```python
from build123d import *

# Parameters (mm, degrees)
F1_DEPTH = 40
F4_DEPTH = 22.7
F6_D     = 3
F6_DEPTH = 5
F6_TIP   = 0.9012909285


with BuildPart() as f1:
    # F0 (on Top) → F1 (new body)
    with BuildSketch(Plane.XY):
        Polygon((16.9819894888, 21.025), (-16.9819894888, 21.025), (-21.025, 16.9819894888), (-21.025, -16.9819894888), (-16.9819894888, -21.025), (16.9819894888, -21.025), (21.025, -16.9819894888), (21.025, 16.9819894888), align=None)
    extrude(amount=-F1_DEPTH)

    # F3 (on offset) + F1_face (on face) → F4 (cut)
    with BuildSketch(Plane.XY.offset(-7.65)):
        Polygon((-21.025, 16.9819894888), (-21.025, 14.5071157546), (-14.5071157546, 21.025), (-16.9819894888, 21.025), align=None)
        Polygon((16.9819894888, 21.025), (14.5071157546, 21.025), (21.025, 14.5071157546), (21.025, 16.9819894888), align=None)
        Polygon((21.025, -14.5071157546), (14.5071157546, -21.025), (16.9819894888, -21.025), (21.025, -16.9819894888), align=None)
        Polygon((-21.025, -16.9819894888), (-16.9819894888, -21.025), (-14.5071157546, -21.025), (-21.025, -14.5071157546), align=None)
    with BuildSketch(Plane(origin=(0, 0, -40), x_dir=(1, 0, 0), z_dir=(0, 0, -1))):
        Polygon((21.025, -16.9819894888), (21.025, 16.9819894888), (16.9819894888, 21.025), (-16.9819894888, 21.025), (-21.025, 16.9819894888), (-21.025, -16.9819894888), (-16.9819894888, -21.025), (16.9819894888, -21.025), align=None)
    extrude(amount=-F4_DEPTH, dir=(0, 0, 1), mode=Mode.SUBTRACT)

    # F6
    with Locations(Plane.XY):
        with Locations((-15.5, 15.5), (15.5, 15.5), (15.5, -15.5), (-15.5, -15.5)):
            Hole(F6_D / 2, depth=F6_DEPTH)
            with Locations((0, 0, -(F6_DEPTH + F6_TIP / 2))):  # 118° drill point
                Cone(0, F6_D / 2, F6_TIP, mode=Mode.SUBTRACT)


solid = f1.part
```
Geometry check sheet. Reference: the model listing, model coordinates, mm. A direction names the side the tool comes from. Give positions to 0.01 mm unless a question says otherwise; leave off trailing zeros. Order: outer loops, then holes, each group sorted by start corner. A loop starts at its lowest first (then second) coordinate and runs counter-clockwise, first axis right, second up.
1. Release check for a two-part mould opening along X. For faces 6 (the face through (18.975, -19.032, -35.107)), 7 (the face through (17, 15.57, -2.54)), 8 (the face through (18, -18, -7.65)) record: pulls with the +X half, pulls with the -X half, needs draft (parallel to the pull), parting line crosses it, or undercut.
2. Gauge pin test, flat end, axial feed: pin 1 Ø6 at (x, y) = (-10.5, 9.5) entering from +Z. Record the tip position at first contact, or that the pin passes through.
3. Thickness scan on L1, parallel to Y at x = -15.5, z = -3.35 (3 decimals); L2, parallel to Y at x = -15, z = -2 (3 decimals). Record the ranges inside material, lowest first.
4. Section check B-B, the plane z = -24. Enter the section's corners in (x, y) (3 decimals), and give its area (3 significant figures).
5. Section check A-A, the plane z = -3. Enter the section's corners in (x, y) (3 decimals), and give its area (3 significant figures).
6. Access from +Z, -Z, +X, -X, +Y, -Y to the whole of each face (thin tool, end or side, straight path). Record for faces 1 (the face through (17.81, -17.72, -18.84)), 2 (the face through (-18.5, 18.5, -30.35)), 3 (the face through (17.72, 17.81, -18.84)), 4 (the face through (-19, -18, -30.35)), 5 (the face through (-14, -15.43, -2.54)).
Values follow:
1. face 6: pulls with the +X half
1. face 7: undercut
1. face 8: needs draft
2. pin 1: stops at z = 0
3. L1: y = -21.025 to -17, -14 to 14, 17 to 21.025
3. L2: y = -21.025 to -16.914, -14.086 to 14.086, 16.914 to 21.025
4. outline: (-21.025, -14.507) - (-14.507, -21.025) - (14.507, -21.025) - (21.025, -14.507) - (21.025, 14.507) - (14.507, 21.025) - (-14.507, 21.025) - (-21.025, 14.507) - close
4. area: 1,680 mm2
5. outline: (-21.025, -16.982) - (-16.982, -21.025) - (16.982, -21.025) - (21.025, -16.982) - (21.025, 16.982) - (16.982, 21.025) - (-16.982, 21.025) - (-21.025, 16.982) - close; hole circle Ø3 at (-15.5, -15.5); hole circle Ø3 at (-15.5, 15.5); hole circle Ø3 at (15.5, -15.5); hole circle Ø3 at (15.5, 15.5)
5. area: 1,710 mm2
6. face 1: +X, -Y
6. face 2: -X, +Y
6. face 3: +X, +Y
6. face 4: -X, -Y
6. face 5: +Z
